```python
from build123d import *

# Parameters (mm, degrees)
SKETCH1_R           = 7.125
BOSS_EXTRUDE1_DEPTH = 4.95
SKETCH2_R           = 4
CUT_EXTRUDE2_DEPTH  = 12.25
CUT_EXTRUDE3_START  = -2.25
SKETCH3_R           = 7.125
SKETCH3_R_2         = 5.998819533
CUT_EXTRUDE3_DEPTH  = 2.25
FILLET1_R           = 0.1
FILLET2_R           = 0.25


with BuildPart() as part:
    # Sketch1 → Boss-Extrude1 (new body)
    with BuildSketch(Plane(origin=(0, 0, 0), x_dir=(1, 0, 0), z_dir=(0, 1, 0))):
        with Locations(Location((0, 0, 0), (0, 0, 90))):
            Circle(SKETCH1_R)
    extrude(amount=BOSS_EXTRUDE1_DEPTH)

    # Sketch2 → Cut-Extrude2 (cut)
    with BuildSketch(Plane(origin=(0, 4.95, 0), x_dir=(1, 0, 0), z_dir=(0, 1, 0))):
        with Locations(Location((0, 0, 0), (0, 0, 270))):
            Circle(SKETCH2_R)
    extrude(amount=-CUT_EXTRUDE2_DEPTH, mode=Mode.SUBTRACT)

    # Sketch3 → Cut-Extrude3 (cut)
    with BuildSketch(Plane(origin=(0, 4.95, 0), x_dir=(1, 0, 0), z_dir=(0, 1, 0)).offset(CUT_EXTRUDE3_START)):
        with Locations(Location((0, 0, 0), (0, 0, 90))):
            Circle(SKETCH3_R)
        with Locations(Location((0, 0, 0), (0, 0, 270))):
            Circle(SKETCH3_R_2, mode=Mode.SUBTRACT)
    extrude(amount=CUT_EXTRUDE3_DEPTH, mode=Mode.SUBTRACT)

    # Fillet1
    fillet1_edges = [part.edges().sort_by_distance(p)[0] for p in [
        (0, 2.7, 7.125),
        (0, 4.95, -5.998819533),
        (0, 0, 7.125),
    ]]
    fillet(fillet1_edges, radius=FILLET1_R)

    # Fillet2
    fillet2_edges = [part.edges().sort_by_distance(p)[0] for p in [
        (0, 0, -4),
        (0, 4.95, -4),
    ]]
    fillet(fillet2_edges, radius=FILLET2_R)


solid = part.part
```
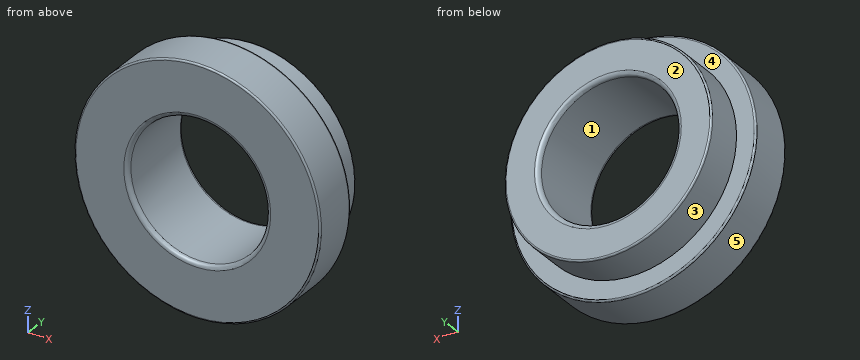
Work out the finished part from the listing and answer in its coordinate system (mm). Face numbers are marked on the shaded views. A direction names the side the tool comes from. Give positions to 0.01 mm unless a question says otherwise; leave off trailing zeros. Loops run counter-clockwise (first coordinate to the right, second up) from the corner with the lowest first, then second, coordinate; pieces in that order, holes last. Notation, with made-up numbers: (58.25, 55.25) -> (81.25, 55.25) arc R35 ccw to (81.25, 92.25) -> close; hole circle Ø8 at (2.5, 58). An arc over 180 degrees is marked (long way). Put each result on its own line as item: value. Start each with the question number.
Item 1: The part is cut by section A-A (z = 0). Give the vertices of the cut face in (x, y) (3 decimals).
Item 2: The part is cut by section B-B (x = 0). Give the vertices of the cut face in (y, z) (3 decimals), then the cut area to 3 significant figures.
Item 3: The mould has two halves that part along Z. Classify the marked faces 1, 2 and 3: released by +Z, released by -Z, zero draft, split by the parting line, or undercut.
Item 4: The part is cut by section D-D (y = 3.6). Give the vertices of the cut face in (x, z).
Item 5: Find the intervals of material crossed by L1, parallel to X at y = 1.6, z = 0 (3 decimals); L2, parallel to X at y = 3.25, z = 0; L3, parallel to Y at x = 1.5, z = 6, in increasing order. Write a range as [from, to].
Item 6: Which of the six approach directions +Z, -Z, +X, -X, +Y, -Y give full straight-line access (tool end or side, diameter ignored) to the marked faces 4 and 5?
Item 7: The part is cut by section C-C (y = 1). Give the vertices of the cut face in (x, z) (3 decimals), then the cut area to 3 significant figures.
Item 8: Each of these flat-tipped pins is pushed along its axis until it touches: P1, Ø2, axis at y = 3, z = 1.5, coming from the +X side; P2, Ø2, axis at x = -5, y = 2, coming from the -Z side. Where does it stop, or does it pass through?
Answers below:
1. outline: (-7.125, 0.1) arc R0.1 ccw to (-7.025, 0) -> (-4.25, 0) arc R0.25 ccw to (-4, 0.25) -> (-4, 4.7) arc R0.25 ccw to (-4.25, 4.95) -> (-5.899, 4.95) arc R0.1 ccw to (-5.999, 4.85) -> (-5.999, 2.7) -> (-7.025, 2.7) arc R0.1 ccw to (-7.125, 2.6) -> close; (4, 0.25) arc R0.25 ccw to (4.25, 0) -> (7.025, 0) arc R0.1 ccw to (7.125, 0.1) -> (7.125, 2.6) arc R0.1 ccw to (7.025, 2.7) -> (5.999, 2.7) -> (5.999, 4.85) arc R0.1 ccw to (5.899, 4.95) -> (4.25, 4.95) arc R0.25 ccw to (4, 4.7) -> close
2. outline: (0, -7.025) arc R0.1 ccw to (0.1, -7.125) -> (2.6, -7.125) arc R0.1 ccw to (2.7, -7.025) -> (2.7, -5.999) -> (4.85, -5.999) arc R0.1 ccw to (4.95, -5.899) -> (4.95, -4.25) arc R0.25 ccw to (4.7, -4) -> (0.25, -4) arc R0.25 ccw to (0, -4.25) -> close; (0, 4.25) arc R0.25 ccw to (0.25, 4) -> (4.7, 4) arc R0.25 ccw to (4.95, 4.25) -> (4.95, 5.899) arc R0.1 ccw to (4.85, 5.999) -> (2.7, 5.999) -> (2.7, 7.025) arc R0.1 ccw to (2.6, 7.125) -> (0.1, 7.125) arc R0.1 ccw to (0, 7.025) -> close
2. area: 25.8 mm2
3. face 1: undercut
3. face 2: zero draft
3. face 3: split by the parting line
4. outline: circle Ø12 at (0, 0); hole circle Ø8 at (0, 0)
5. L1: [-7.125, -4], [4, 7.125]
5. L2: [-6, -4], [4, 6]
5. L3: [0, 2.7]
6. face 4: +Y
6. face 5: +Y, -Y
7. outline: circle Ø14.25 at (0, 0); hole circle Ø8 at (0, 0)
7. area: 109 mm2
8. P1: x = 7.1
8. P2: z = -5.9
